```python
from build123d import *

# Parameters (mm, degrees)
SKETCH1_W           = 25.4
SKETCH1_H           = 1397
SKETCH1_R           = 3.175
BOSS_EXTRUDE1_DEPTH = 3.175
SKETCH2_W           = 25.4
SKETCH2_H           = 546.210923287
CUT_EXTRUDE1_DEPTH  = 699.622659685


with BuildPart() as part:
    # Sketch1 → Boss-Extrude1 (new body)
    with BuildSketch(Plane(origin=(0, 0, 0), x_dir=(0, 0, -1), z_dir=(1, 0, 0))):
        Rectangle(SKETCH1_W, SKETCH1_H)
        with Locations((0, -685.8)):
            Circle(SKETCH1_R, mode=Mode.SUBTRACT)
        with Locations((0, -673.1)):
            Circle(SKETCH1_R, mode=Mode.SUBTRACT)
        with Locations((0, -660.4)):
            Circle(SKETCH1_R, mode=Mode.SUBTRACT)
        with Locations((0, -647.7)):
            Circle(SKETCH1_R, mode=Mode.SUBTRACT)
        with Locations((0, -635)):
            Circle(SKETCH1_R, mode=Mode.SUBTRACT)
        with Locations((0, -622.3)):
            Circle(SKETCH1_R, mode=Mode.SUBTRACT)
        with Locations((0, -609.6)):
            Circle(SKETCH1_R, mode=Mode.SUBTRACT)
        with Locations((0, -596.9)):
            Circle(SKETCH1_R, mode=Mode.SUBTRACT)
        with Locations((0, -584.2)):
            Circle(SKETCH1_R, mode=Mode.SUBTRACT)
        with Locations((0, -571.5)):
            Circle(SKETCH1_R, mode=Mode.SUBTRACT)
        with Locations((0, -558.8)):
            Circle(SKETCH1_R, mode=Mode.SUBTRACT)
        with Locations((0, -546.1)):
            Circle(SKETCH1_R, mode=Mode.SUBTRACT)
        with Locations((0, -533.4)):
            Circle(SKETCH1_R, mode=Mode.SUBTRACT)
        with Locations((0, -520.7)):
            Circle(SKETCH1_R, mode=Mode.SUBTRACT)
        with Locations((0, -508)):
            Circle(SKETCH1_R, mode=Mode.SUBTRACT)
        with Locations((0, -495.3)):
            Circle(SKETCH1_R, mode=Mode.SUBTRACT)
        with Locations((0, -482.6)):
            Circle(SKETCH1_R, mode=Mode.SUBTRACT)
        with Locations((0, -469.9)):
            Circle(SKETCH1_R, mode=Mode.SUBTRACT)
        with Locations((0, -457.2)):
            Circle(SKETCH1_R, mode=Mode.SUBTRACT)
        with Locations((0, -444.5)):
            Circle(SKETCH1_R, mode=Mode.SUBTRACT)
        with Locations((0, -431.8)):
            Circle(SKETCH1_R, mode=Mode.SUBTRACT)
        with Locations((0, -419.1)):
            Circle(SKETCH1_R, mode=Mode.SUBTRACT)
        with Locations((0, -406.4)):
            Circle(SKETCH1_R, mode=Mode.SUBTRACT)
        with Locations((0, -393.7)):
            Circle(SKETCH1_R, mode=Mode.SUBTRACT)
        with Locations((0, -381)):
            Circle(SKETCH1_R, mode=Mode.SUBTRACT)
        with Locations((0, -368.3)):
            Circle(SKETCH1_R, mode=Mode.SUBTRACT)
        with Locations((0, -355.6)):
            Circle(SKETCH1_R, mode=Mode.SUBTRACT)
        with Locations((0, -342.9)):
            Circle(SKETCH1_R, mode=Mode.SUBTRACT)
        with Locations((0, -330.2)):
            Circle(SKETCH1_R, mode=Mode.SUBTRACT)
        with Locations((0, -317.5)):
            Circle(SKETCH1_R, mode=Mode.SUBTRACT)
        with Locations((0, -304.8)):
            Circle(SKETCH1_R, mode=Mode.SUBTRACT)
        with Locations((0, -292.1)):
            Circle(SKETCH1_R, mode=Mode.SUBTRACT)
        with Locations((0, -279.4)):
            Circle(SKETCH1_R, mode=Mode.SUBTRACT)
        with Locations((0, -266.7)):
            Circle(SKETCH1_R, mode=Mode.SUBTRACT)
        with Locations((0, -254)):
            Circle(SKETCH1_R, mode=Mode.SUBTRACT)
        with Locations((0, -241.3)):
            Circle(SKETCH1_R, mode=Mode.SUBTRACT)
        with Locations((0, -228.6)):
            Circle(SKETCH1_R, mode=Mode.SUBTRACT)
        with Locations((0, -215.9)):
            Circle(SKETCH1_R, mode=Mode.SUBTRACT)
        with Locations((0, -203.2)):
            Circle(SKETCH1_R, mode=Mode.SUBTRACT)
        with Locations((0, -190.5)):
            Circle(SKETCH1_R, mode=Mode.SUBTRACT)
        with Locations((0, -177.8)):
            Circle(SKETCH1_R, mode=Mode.SUBTRACT)
        with Locations((0, -165.1)):
            Circle(SKETCH1_R, mode=Mode.SUBTRACT)
        with Locations((0, -152.4)):
            Circle(SKETCH1_R, mode=Mode.SUBTRACT)
        with Locations((0, -139.7)):
            Circle(SKETCH1_R, mode=Mode.SUBTRACT)
        with Locations((0, -127)):
            Circle(SKETCH1_R, mode=Mode.SUBTRACT)
        with Locations((0, -114.3)):
            Circle(SKETCH1_R, mode=Mode.SUBTRACT)
        with Locations((0, -101.6)):
            Circle(SKETCH1_R, mode=Mode.SUBTRACT)
        with Locations((0, -88.9)):
            Circle(SKETCH1_R, mode=Mode.SUBTRACT)
        with Locations((0, -76.2)):
            Circle(SKETCH1_R, mode=Mode.SUBTRACT)
        with Locations((0, -63.5)):
            Circle(SKETCH1_R, mode=Mode.SUBTRACT)
        with Locations((0, -50.8)):
            Circle(SKETCH1_R, mode=Mode.SUBTRACT)
        with Locations((0, -38.1)):
            Circle(SKETCH1_R, mode=Mode.SUBTRACT)
        with Locations((0, -25.4)):
            Circle(SKETCH1_R, mode=Mode.SUBTRACT)
        with Locations((0, -12.7)):
            Circle(SKETCH1_R, mode=Mode.SUBTRACT)
        Circle(SKETCH1_R, mode=Mode.SUBTRACT)
        with Locations((0, 12.7)):
            Circle(SKETCH1_R, mode=Mode.SUBTRACT)
        with Locations((0, 25.4)):
            Circle(SKETCH1_R, mode=Mode.SUBTRACT)
        with Locations((0, 38.1)):
            Circle(SKETCH1_R, mode=Mode.SUBTRACT)
        with Locations((0, 50.8)):
            Circle(SKETCH1_R, mode=Mode.SUBTRACT)
        with Locations((0, 63.5)):
            Circle(SKETCH1_R, mode=Mode.SUBTRACT)
        with Locations((0, 76.2)):
            Circle(SKETCH1_R, mode=Mode.SUBTRACT)
        with Locations((0, 88.9)):
            Circle(SKETCH1_R, mode=Mode.SUBTRACT)
        with Locations((0, 101.6)):
            Circle(SKETCH1_R, mode=Mode.SUBTRACT)
        with Locations((0, 114.3)):
            Circle(SKETCH1_R, mode=Mode.SUBTRACT)
        with Locations((0, 127)):
            Circle(SKETCH1_R, mode=Mode.SUBTRACT)
        with Locations((0, 139.7)):
            Circle(SKETCH1_R, mode=Mode.SUBTRACT)
        with Locations((0, 152.4)):
            Circle(SKETCH1_R, mode=Mode.SUBTRACT)
        with Locations((0, 165.1)):
            Circle(SKETCH1_R, mode=Mode.SUBTRACT)
        with Locations((0, 177.8)):
            Circle(SKETCH1_R, mode=Mode.SUBTRACT)
        with Locations((0, 190.5)):
            Circle(SKETCH1_R, mode=Mode.SUBTRACT)
        with Locations((0, 203.2)):
            Circle(SKETCH1_R, mode=Mode.SUBTRACT)
        with Locations((0, 215.9)):
            Circle(SKETCH1_R, mode=Mode.SUBTRACT)
        with Locations((0, 228.6)):
            Circle(SKETCH1_R, mode=Mode.SUBTRACT)
        with Locations((0, 241.3)):
            Circle(SKETCH1_R, mode=Mode.SUBTRACT)
        with Locations((0, 254)):
            Circle(SKETCH1_R, mode=Mode.SUBTRACT)
        with Locations((0, 266.7)):
            Circle(SKETCH1_R, mode=Mode.SUBTRACT)
        with Locations((0, 279.4)):
            Circle(SKETCH1_R, mode=Mode.SUBTRACT)
        with Locations((0, 292.1)):
            Circle(SKETCH1_R, mode=Mode.SUBTRACT)
        with Locations((0, 304.8)):
            Circle(SKETCH1_R, mode=Mode.SUBTRACT)
        with Locations((0, 317.5)):
            Circle(SKETCH1_R, mode=Mode.SUBTRACT)
        with Locations((0, 330.2)):
            Circle(SKETCH1_R, mode=Mode.SUBTRACT)
        with Locations((0, 342.9)):
            Circle(SKETCH1_R, mode=Mode.SUBTRACT)
        with Locations((0, 355.6)):
            Circle(SKETCH1_R, mode=Mode.SUBTRACT)
        with Locations((0, 368.3)):
            Circle(SKETCH1_R, mode=Mode.SUBTRACT)
        with Locations((0, 381)):
            Circle(SKETCH1_R, mode=Mode.SUBTRACT)
        with Locations((0, 393.7)):
            Circle(SKETCH1_R, mode=Mode.SUBTRACT)
        with Locations((0, 406.4)):
            Circle(SKETCH1_R, mode=Mode.SUBTRACT)
        with Locations((0, 419.1)):
            Circle(SKETCH1_R, mode=Mode.SUBTRACT)
        with Locations((0, 431.8)):
            Circle(SKETCH1_R, mode=Mode.SUBTRACT)
        with Locations((0, 444.5)):
            Circle(SKETCH1_R, mode=Mode.SUBTRACT)
        with Locations((0, 457.2)):
            Circle(SKETCH1_R, mode=Mode.SUBTRACT)
        with Locations((0, 469.9)):
            Circle(SKETCH1_R, mode=Mode.SUBTRACT)
        with Locations((0, 482.6)):
            Circle(SKETCH1_R, mode=Mode.SUBTRACT)
        with Locations((0, 495.3)):
            Circle(SKETCH1_R, mode=Mode.SUBTRACT)
        with Locations((0, 508)):
            Circle(SKETCH1_R, mode=Mode.SUBTRACT)
        with Locations((0, 520.7)):
            Circle(SKETCH1_R, mode=Mode.SUBTRACT)
        with Locations((0, 533.4)):
            Circle(SKETCH1_R, mode=Mode.SUBTRACT)
        with Locations((0, 546.1)):
            Circle(SKETCH1_R, mode=Mode.SUBTRACT)
        with Locations((0, 558.8)):
            Circle(SKETCH1_R, mode=Mode.SUBTRACT)
        with Locations((0, 571.5)):
            Circle(SKETCH1_R, mode=Mode.SUBTRACT)
        with Locations((0, 584.2)):
            Circle(SKETCH1_R, mode=Mode.SUBTRACT)
        with Locations((0, 596.9)):
            Circle(SKETCH1_R, mode=Mode.SUBTRACT)
        with Locations((0, 609.6)):
            Circle(SKETCH1_R, mode=Mode.SUBTRACT)
        with Locations((0, 622.3)):
            Circle(SKETCH1_R, mode=Mode.SUBTRACT)
        with Locations((0, 635)):
            Circle(SKETCH1_R, mode=Mode.SUBTRACT)
        with Locations((0, 647.7)):
            Circle(SKETCH1_R, mode=Mode.SUBTRACT)
        with Locations((0, 660.4)):
            Circle(SKETCH1_R, mode=Mode.SUBTRACT)
        with Locations((0, 673.1)):
            Circle(SKETCH1_R, mode=Mode.SUBTRACT)
        with Locations((0, 685.8)):
            Circle(SKETCH1_R, mode=Mode.SUBTRACT)
    extrude(amount=BOSS_EXTRUDE1_DEPTH)

    # Sketch2 → Cut-Extrude1 (cut, through all)
    with BuildSketch(Plane.ZY):
        with Locations((0, 425.394538356)):
            Rectangle(SKETCH2_W, SKETCH2_H)
    extrude(amount=-CUT_EXTRUDE1_DEPTH, mode=Mode.SUBTRACT)


solid = part.part
```
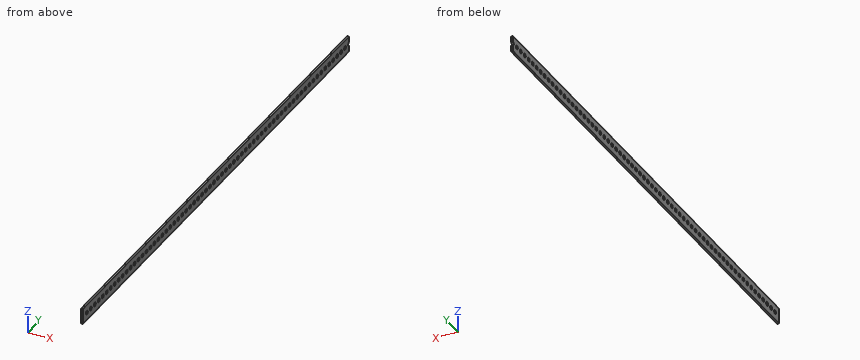
For this review, take the finished solid that the model builds, in its own axes (mm). Coordinates: 2 decimals unless noted, no trailing zeros. Use one line per item in the form item = value. Start each with the question number.
1) Take a section at A-A (x = 1.2). State how many separate pieces and enclosed holes the cut face has, plus the area to 3 significant figures.
2) For pin 1 (8.5 mm diameter, centred on y = 76.2, z = 0, fed in from -X); pin 2 (1.5 mm diameter, centred on x = 2.5, z = 0.5, fed in from +Y), all flat-tipped, find the tip position at first contact; note any pin that passes through.
3) To check wall thickness, follow probe 1 along Z at (x, y) = (1.8, -152.4) (3 decimals); probe 2 along Z at (x, y) = (0.2, -472). State the ranges of each line that lie inside material, in increasing order. Write a range as from..to.
From the geometry:
q1.separate_pieces = 1
q1.enclosed_holes = 66
q1.area = 19,500 mm2
q2.pin_1 = 0
q2.pin_2 = 149.48
q3.probe_1 = -12.7..-3.175, 3.175..12.7
q3.probe_2 = -12.7..-2.38, 2.38..12.7
